Autodesk Inventor part; units mm, degrees
ref_plane "YZ Plane" through (0, 0, 0) normal (1, 0, 0) x (0, 1, 0)
ref_plane "XZ Plane" through (0, 0, 0) normal (0, 1, 0) x (-1, 0, 0)
ref_plane "XY Plane" through (0, 0, 0) normal (0, 0, 1) x (1, 0, 0)
sketch "Sketch2" plane through (0, 0, 0) normal (0, 0, 1) x (1, 0, 0)
  line L0 (-12.5, -16.8475) -> (-12.5, -10.7194)
  line L1 (12.5, -12.5194) -> (12.5, -16.8475)
  line L2 (12.5, -20) -> (-12.5, 20) construction
  line L3 (-12.5, -20) -> (12.5, 20) construction
  arc A0 (12.5, 20) -> (-12.5, 20) centre (0, 20) ccw
  arc A1 (-23.9938, -6.3332) -> (-26.3611, -9.6367) centre (-26.3611, -7.1367) ccw
  arc A2 (-21.3611, 3.8099) -> (-23.8611, 1.3099) centre (-23.8611, 3.8099) ccw
  arc A3 (-21.3611, -18.5591) -> (-25.4614, -20.4798) centre (-23.8611, -18.5591) ccw
  arc A4 (22.9392, 3.8099) -> (18.0516, 3.0686) centre (20.4392, 3.8099) ccw
  arc A5 (30.6335, -7.1367) -> (25.6339, -7.1814) centre (28.1335, -7.1367) ccw
  arc A6 (21.1908, -24.646) -> (17.9392, -20.8491) centre (19.6037, -22.7144) ccw
  spline S0 degree 2 poles (-23.8611, 1.3099) (-19.0526, -6.9708) (-12.5, -10.7194) knots 0 0 0 1 1 1
  spline S1 degree 2 poles (-21.3611, 3.8099) (-18.5864, -3.6522) (-12.5, -6.6832) knots 0 0 0 1 1 1
  spline S2 degree 2 poles (-26.3611, -9.6367) (-21.4971, -18.1116) (-12.5, -20) knots 0 0 0 1 1 1
  spline S3 degree 2 poles (-24.0407, -6.2062) (-21.0395, -14.4004) (-12.5, -16.8475) knots 0 0 0 1 1 1
  spline S4 degree 2 poles (-21.3611, -18.5591) (-18.1547, -28.3248) (-10.356, -20) knots 0 0 0 1 1 1
  spline S5 degree 2 poles (-25.4614, -20.4798) (-20.4927, -34.7918) (-6.9898, -20) knots 0 0 0 1 1 1
  spline S6 degree 2 poles (17.9392, 3.8099) (20.0689, -9.5172) (12.5, -9.6367) knots 0 0 0 1 1 1
  spline S7 degree 2 poles (22.9392, 3.8099) (24.5184, -8.2792) (12.5, -12.5194) knots 0 0 0 1 1 1
  spline S8 degree 2 poles (25.8131, -6.2062) (24.8315, -13.7331) (12.5, -16.8475) knots 0 0 0 1 1 1
  spline S9 degree 2 poles (30.6335, -7.1367) (30.4955, -17.6904) (12.5, -20) knots 0 0 0 1 1 1
  spline S10 degree 2 poles (9.1202, -20) (9.7376, -27.3779) (17.9392, -20.8491) knots 0 0 0 1 1 1
  spline S11 degree 3 poles (21.1908, -24.646) (15.8936, -29.7076) (6.4999, -29.4415) (5.3692, -20) knots 0 0 0 0 1 1 1 1
  spline S12 degree 2 poles (12.5, 20) (7.4894, -0.1647) (12.5, -9.6367) knots 0 0 0 1 1 1
  spline S13 degree 2 poles (-12.5, 20) (-7.9354, -0.2578) (-12.5, -6.6832) knots 0 0 0 1 1 1
  line L4 (12.5, -20) -> (9.1202, -20)
  line L5 (-10.356, -20) -> (-12.5, -20)
  spline S14 degree 2 poles (-6.9898, -20) (0.0212, -17.9924) (5.3692, -20) knots 0 0 0 1 1 1
  point P0 (0, 0)
  point P1 (-18.2659, -6.203)
  point P2 (-17.5697, -2.7642)
  point P3 (-20.3482, -16.5508)
  point P4 (-19.6835, -12.9372)
  point P5 (-17.232, -23.7647)
  point P6 (-19.3511, -27.4539)
  point P7 (17.0045, -7.4262)
  point P8 (21.1905, -6.2037)
  point P9 (22.9403, -11.7957)
  point P10 (27.4494, -14.4708)
  point P11 (11.0482, -23.7717)
  point P12 (14.8952, -27.8035)
  point P13 (9.1239, -26.7454)
  point P14 (10.0714, -0.0017)
  point P15 (-10.3694, -0.0099)
  point P16 (0, -19.0003)
  dimension "d6" = 40
  dimension "d7" = 25
  dimension "d8" = 5
  dimension "d9" = 5
  dimension "d10" = 5
  dimension "d11" = 5
  dimension "d12" = 5
  dimension "d13" = 5
extrude "Extrusion1" add sketch "Sketch2" along normal blind 10 contours L0 S0 A2 S1 S13 A0 S12 S6 A4 S7 L1 S8 A5 S9 L4 S10 A6 S11 S14 S5 A3 S4 L5 S2 A1 S3
sketch "Sketch3" plane through (0, 0, 0) normal (0, 0, -1) x (-1, 0, 0)
  line L0 (7.5, -10) -> (-7.5, -10)
  line L1 (-7.5, -10) -> (-7.5, 10)
  line L2 (-7.5, 10) -> (7.5, 10)
  line L3 (7.5, 10) -> (7.5, -10)
  line L4 (7.5, -10) -> (-7.5, 10) construction
  line L5 (-7.5, -10) -> (7.5, 10) construction
  point P0 (0, 0)
  dimension "d16" = 15
  dimension "d17" = 20
extrude "Belt box" add sketch "Sketch3" along normal blind 15
sketch "Sketch4" plane through (0, 0, -15) normal (0, 0, -1) x (-1, 0, 0)
  line L0 (0, 0) -> (0, 8) construction
  line L1 (0, 0) -> (0, -8) construction
  line L2 (7.5, 7.65) -> (-7.5, 7.65)
  line L3 (-7.5, 7.65) -> (-7.5, 8.35)
  line L4 (-7.5, 8.35) -> (7.5, 8.35)
  line L5 (7.5, 8.35) -> (7.5, 7.65)
  line L6 (7.5, 7.65) -> (-7.5, 8.35) construction
  line L7 (-7.5, 7.65) -> (7.5, 8.35) construction
  line L8 (7.5, -21.75) -> (-7.5, -21.75)
  line L9 (-7.5, -21.75) -> (-7.5, 5.75)
  line L10 (-7.5, 5.75) -> (7.5, 5.75)
  line L11 (7.5, 5.75) -> (7.5, -21.75)
  line L12 (7.5, -21.75) -> (-7.5, 5.75) construction
  line L13 (-7.5, -21.75) -> (7.5, 5.75) construction
  dimension "d20" = 8
  dimension "d21" = 8
  dimension "d22" = 15
  dimension "d23" = 0.7
  dimension "d24" = 15
  dimension "d25" = 27.5
extrude "belt cut out" cut sketch "Sketch4" against normal blind 15
sketch "Sketch5" plane through (0, 0, 10) normal (0, 0, 1) x (1, 0, 0)
  line L0 (-17.5, 33) -> (17.5, 33)
  line L1 (20, 33) -> (20, 32)
  line L2 (20, 32) -> (-20, 32)
  line L3 (-20, 32) -> (-20, 33)
  arc A0 (12.5, 20) -> (-12.5, 20) centre (0, 20) ccw
  line L4 (-20, 33) -> (20, 32) construction
  line L5 (20, 33) -> (-20, 32) construction
  line L6 (-20, 33) -> (-20, 58) construction
  line L7 (20, 33) -> (20, 58) construction
  line L8 (-20, 33) -> (-20, 41)
  line L9 (-20, 41) -> (-17.5, 41)
  line L10 (-17.5, 41) -> (-17.5, 33)
  line L11 (20, 33) -> (20, 41)
  line L12 (20, 41) -> (17.5, 41)
  line L13 (17.5, 41) -> (17.5, 33)
  point P0 (0, 0)
  point P1 (0, 32.5)
  point P2 (-3.5, 32)
  point P3 (3.5, 32)
  dimension "d29" = 1
  dimension "d30" = 25
  dimension "d31" = 25
  dimension "d33" = 8
  dimension "d34" = 8
extrude "Extrusion4" add sketch "Sketch5" against normal blind 10 contours L0 L13 L12 L11 L1 L2 A0 L3 L8 L9 L10
properties part number "octopus_on_belt"
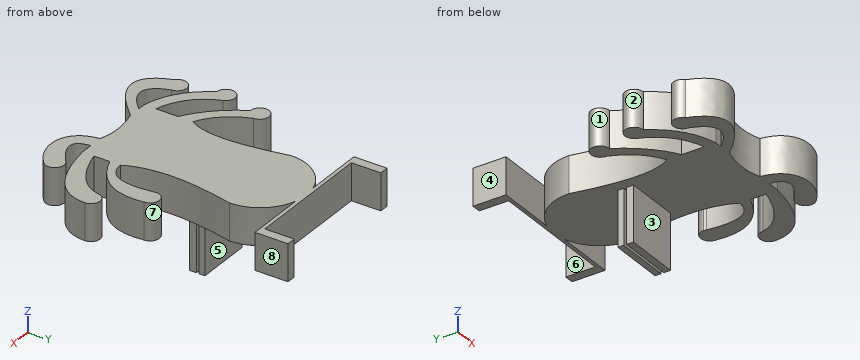
Input: part model. Units: mm. Frame: model coordinates. Face numbers are marked on the shaded views. A direction names the side the tool comes from. Coordinates: 2 decimals unless noted, no trailing zeros. Write each loop counter-clockwise with the first axis right and the second up, starting at its lowest first coordinate (ties: lowest second). Pieces come first, ordered by that corner, then holes.
1) Pin query (flat end, axial travel): pin 1 Ø3 at (x, z) = (5.5, -3.5) entering from +Y; pin 2 Ø5 at (y, z) = (-12.5, 6) entering from -X; pin 3 Ø11 at (x, z) = (-2.5, 5) entering from +Y; pin 4 Ø12 at (x, y) = (2.5, 13) entering from -Z. Return the tip coordinate at first contact, or that it passes through.
2) Section C-C on x = 15.5. State how many separate pieces and enclosed holes the cut face has, and give its area (3 significant figures).
3) Section D-D on y = 24.5. Output: boundary loops of the cut face in (x, z), and give its area (3 significant figures).
4) Section B-B on y = 35. Output: boundary loops of the cut face in (x, z).
5) Set-up query: the marked faces 5, 6, 7 and 8. Return all of +Z, -Z, +X, -X, +Y, -Y with unobstructed straight access to the full face (end or side cutting, diameter ignored); none if empty.
6) Mould query, pull axis X, two halves, no side actions, for the marked faces 1, 2, 3 and 4. Classes: pulls with the +X half, pulls with the -X half, needs draft (parallel to the pull), parting line crosses it, or undercut.
7) Section A-A on z = -2. Output: boundary loops of the cut face in (x, y), and give its area (4 significant figures).
8) Material intervals for line 1 along Y through (x, z) = (7, -9.5); line 2 along X through (y, z) = (34.5, 6.5); line 3 along X through (y, z) = (-23, 0.75), sorted ascending.
Check result:
1. pin 1: stops at y = 10
1. pin 2: stops at x = -26.15
1. pin 3: stops at y = 33
1. pin 4: stops at z = -15
2. separate pieces: 4
2. enclosed holes: 0
2. area: 120 mm2
3. outline: (-11.66, 0) - (11.66, 0) - (11.66, 10) - (-11.66, 10) - close
3. area: 233 mm2
4. outline: (-20, 0) - (-17.5, 0) - (-17.5, 10) - (-20, 10) - close; (17.5, 0) - (20, 0) - (20, 10) - (17.5, 10) - close
5. face 5: -Z, +X, -X, +Y
5. face 6: +Z, -Z, +Y
5. face 7: +Z, -Z
5. face 8: +Z, -Z, +X, +Y
6. face 1: undercut
6. face 2: undercut
6. face 3: needs draft
6. face 4: pulls with the -X half
7. outline: (-7.5, 5.75) - (7.5, 5.75) - (7.5, 7.65) - (-7.5, 7.65) - close; (-7.5, 8.35) - (7.5, 8.35) - (7.5, 10) - (-7.5, 10) - close
7. area: 53.25 mm2
8. line 1: y = 5.75 to 7.65, 8.35 to 10
8. line 2: x = -20 to -17.5, 17.5 to 20
8. line 3: x = -24.41 to -18.79, -13.91 to -9.96, 6.11 to 10.03, 14.79 to 22.09
